Geometry: final body of the model. Coordinates: model frame, mm. A direction names the side the tool comes from. Coordinates: 2 decimals unless noted, no trailing zeros. Order: outer loops, then holes, each group sorted by start corner. A loop starts at its lowest first (then second) coordinate and runs counter-clockwise, first axis right, second up. Notation, with made-up numbers: (4, 36.5) - (32, 36.5) arc R14 ccw to (32, 52.5) - close; hole circle Ø3 at (59, -39). An arc over 180 degrees is marked (long way). Use a Markdown table: item, result. Add a question column.
```python
from build123d import *

# Parameters (mm, degrees)
F0_W     = 107.95
F0_H     = 120.65
F0_R     = 3.175
F0_R_2   = 20.32
F1_DEPTH = 8.89


with BuildPart() as f1:
    # F0 (on Top) → F1 (new body)
    with BuildSketch(Plane.XY):
        with Locations((53.975, -60.325)):
            Rectangle(F0_W, F0_H)
        with Locations((11.43, -58.931326)):
            Circle(F0_R, mode=Mode.SUBTRACT)
        with Locations((20.32, -58.931326)):
            Circle(F0_R, mode=Mode.SUBTRACT)
        with Locations((29.21, -58.931326)):
            Circle(F0_R, mode=Mode.SUBTRACT)
        with Locations((38.1, -58.931326)):
            Circle(F0_R, mode=Mode.SUBTRACT)
        with BuildLine():
            ThreePointArc((53.34, -19.05), (57.059744, -10.069744), (66.04, -6.35))
            Line((66.04, -6.35), (88.9, -6.35))
            ThreePointArc((88.9, -6.35), (97.880256, -10.069744), (101.6, -19.05))
            Line((101.6, -19.05), (101.6, -101.6))
            ThreePointArc((101.6, -101.6), (97.880256, -110.580256), (88.9, -114.3))
            Line((88.9, -114.3), (53.34, -114.3))
            Line((53.34, -114.3), (52.828665, -114.3))
            Line((52.828665, -114.3), (19.05, -114.3))
            ThreePointArc((19.05, -114.3), (10.069744, -110.580256), (6.35, -101.6))
            Line((6.35, -101.6), (6.35, -80.521326))
            ThreePointArc((6.35, -80.521326), (10.069744, -71.54107), (19.05, -67.821326))
            Line((19.05, -67.821326), (53.34, -67.821326))
            Line((53.34, -67.821326), (53.34, -19.05))
        make_face(mode=Mode.SUBTRACT)
        with Locations((26.67, -26.67)):
            Circle(F0_R_2, mode=Mode.SUBTRACT)
    extrude(amount=F1_DEPTH)


solid = f1.part
```
1) Access query for faces 5 (the flat face through (50, -51, 8.89)), 6 (the cylindrical face through (97.98, -110.48, 4.38)). Directions: +Z, -Z, +X, -X, +Y, -Y. A direction counts if a zero-diameter tool reaches every point of the face in a straight line with its end or side. Return the directions, or none.
2) Section query C-C (y = -110). Return the cut outline in (x, z).
3) Section query D-D (z = 2). Return the cut outline in (x, y) (3 decimals), and give its area (3 significant figures).
4) Line query: line 1 (X direction, y = -59, z = 2); line 2 (X direction, y = -93, z = 5.5); line 3 (X direction, y = -48, z = 0.5). Output: solid intervals per line, ascending. Write a range as from..to.
5) Section query B-B (y = -26.67). Return the cut outline in (x, z).
6) Draft query along X for faces 1 (the cylindrical face through (10.17, -110.68, 4.38)), 2 (the flat face through (0, -61, 4)), 3 (the flat face through (77, -6.35, 4)), 4 (the flat face through (53, -120.65, 4)). Return one class per face: released by +X, released by -X, zero draft, split by the parting line, or undercut.
7) Section query A-A (x = 49.5). Return the cut outline in (y, z), and give its area (3 significant figures).
From the geometry:
| question | item | result |
|---|---|---|
| 1 | face 5 | +Z, +X, -X, +Y, -Y |
| 1 | face 6 | +Z, -Z |
| 2 | outline | (0, 0) - (9.52, 0) - (9.52, 8.89) - (0, 8.89) - close; (98.43, 0) - (107.95, 0) - (107.95, 8.89) - (98.43, 8.89) - close |
| 3 | outline | (0, -120.65) - (107.95, -120.65) - (107.95, 0) - (0, 0) - close; hole (6.35, -101.6) arc R12.7 ccw to (19.05, -114.3) - (88.9, -114.3) arc R12.7 ccw to (101.6, -101.6) - (101.6, -19.05) arc R12.7 ccw to (88.9, -6.35) - (66.04, -6.35) arc R12.7 ccw to (53.34, -19.05) - (53.34, -67.821) - (19.05, -67.821) arc R12.7 ccw to (6.35, -80.521) - close; hole circle Ø40.64 at (26.67, -26.67); hole circle Ø6.35 at (11.43, -58.931); hole circle Ø6.35 at (20.32, -58.931); hole circle Ø6.35 at (29.21, -58.931); hole circle Ø6.35 at (38.1, -58.931) |
| 3 | area | 4,380 mm^2 |
| 4 | line 1 | x = 0..8.26, 14.6..17.15, 23.49..26.04, 32.38..34.93, 41.27..53.34, 101.6..107.95 |
| 4 | line 2 | x = 0..6.35, 101.6..107.95 |
| 4 | line 3 | x = 0..53.34, 101.6..107.95 |
| 5 | outline | (0, 0) - (6.35, 0) - (6.35, 8.89) - (0, 8.89) - close; (46.99, 0) - (53.34, 0) - (53.34, 8.89) - (46.99, 8.89) - close; (101.6, 0) - (107.95, 0) - (107.95, 8.89) - (101.6, 8.89) - close |
| 6 | face 1 | undercut |
| 6 | face 2 | released by -X |
| 6 | face 3 | undercut |
| 6 | face 4 | zero draft |
| 7 | outline | (-120.65, 0) - (-114.3, 0) - (-114.3, 8.89) - (-120.65, 8.89) - close; (-67.82, 0) - (0, 0) - (0, 8.89) - (-67.82, 8.89) - close |
| 7 | area | 659 mm^2 |
